```python
from build123d import *

# Parameters (mm, degrees)
SKETCH_1_R      = 20
SKETCH_1_R_2    = 5
SKETCH_1_R_3    = 1.5
EXTRUDE_1_DEPTH = 5


with BuildPart() as part:
    # 草圖1 → 填料-伸長1 (new body)
    with BuildSketch(Plane.XY):
        Circle(SKETCH_1_R)
        Circle(SKETCH_1_R_2, mode=Mode.SUBTRACT)
        with Locations((-10, -10)):
            Circle(SKETCH_1_R_3, mode=Mode.SUBTRACT)
        with Locations(Location((-10, 10, 0), (0, 0, 180))):
            Circle(SKETCH_1_R_3, mode=Mode.SUBTRACT)
        with Locations((10, 10)):
            Circle(SKETCH_1_R_3, mode=Mode.SUBTRACT)
        with Locations(Location((10, -10, 0), (0, 0, 180))):
            Circle(SKETCH_1_R_3, mode=Mode.SUBTRACT)
    extrude(amount=EXTRUDE_1_DEPTH)


solid = part.part
```
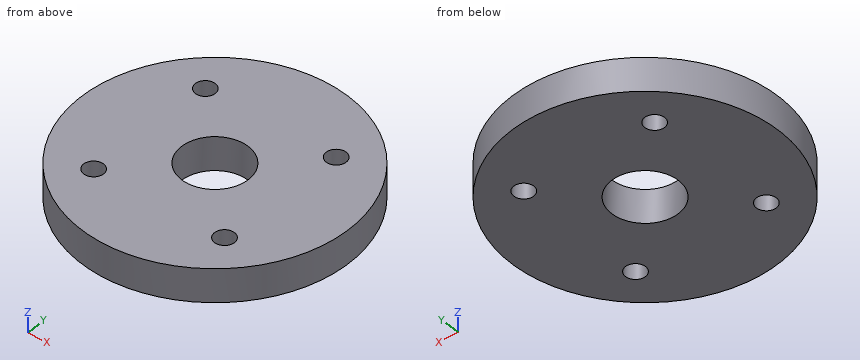
Could you check a few things on this model? Use its own coordinates, in mm. Round coordinates to 2 decimals unless told otherwise and drop trailing zeros. Loops run counter-clockwise (first coordinate to the right, second up) from the corner with the lowest first, then second, coordinate; pieces in that order, holes last. Notation, with made-up numbers: (-19.5, -30) - (38.5, -30) arc R10 ccw to (38.5, -20) - close; hole circle Ø11 at (79, 18.5). An arc over 180 degrees is marked (long way). Use CSV: the item, a comma, the result in double quotes.
Item 1: I need wall thicknesses on L1, parallel to Y at x = 0, z = 1.3; L2, parallel to Y at x = -10, z = 1.95; L3, parallel to X at y = -9, z = 1.15. Which ranges of each line are inside material? Lowest first, please. Write a range as [from, to].
Here are the results:
L1,"y = [-20, -5], [5, 20]"
L2,"y = [-17.32, -11.5], [-8.5, 8.5], [11.5, 17.32]"
L3,"x = [-17.86, -11.12], [-8.88, 8.88], [11.12, 17.86]"
Item 2: If we section it at A-A on y = 0: List the corners of the cut face in (x, z) for me, then the cut area to 3 significant figures.
Here are the results:
outline,"(-20, 0) - (-5, 0) - (-5, 5) - (-20, 5) - close; (5, 0) - (20, 0) - (20, 5) - (5, 5) - close"
area,"150 mm²"
Item 3: Will these pins go through, and if not, where does the flat tip stop? pin 1 (4 mm diameter, centred on x = 10, y = 10, fed in from -Z); pin 2 (1 mm diameter, centred on x = 14.5, z = 1, fed in from -Y); pin 3 (1 mm diameter, centred on x = -1, z = 3.5, fed in from -Y).
Here are the results:
pin 1,"stops at z = 0"
pin 2,"stops at y = -14.28"
pin 3,"stops at y = -19.99"
Item 4: If we section it at D-D on x = 10: List the corners of the cut face in (y, z) for me, then the cut area to 3 significant figures.
Here are the results:
outline,"(-17.32, 0) - (-11.5, 0) - (-11.5, 5) - (-17.32, 5) - close; (-8.5, 0) - (8.5, 0) - (8.5, 5) - (-8.5, 5) - close; (11.5, 0) - (17.32, 0) - (17.32, 5) - (11.5, 5) - close"
area,"143 mm²"
Item 5: If we section it at C-C on z = 2.75: List the corners of the cut face in (x, y) for me, then the cut area to 3 significant figures.
Here are the results:
outline,"circle Ø40 at (0, 0); hole circle Ø3 at (-10, -10); hole circle Ø3 at (-10, 10); hole circle Ø10 at (0, 0); hole circle Ø3 at (10, -10); hole circle Ø3 at (10, 10)"
area,"1,150 mm²"
